Answer from the drawing. Dimensions are ordinates in mm from the lowest x, y and z of the part. A direction names the side the tool comes from. Round coordinates to 2 decimals unless told otherwise and drop trailing zeros. Loops run counter-clockwise (first coordinate to the right, second up) from the corner with the lowest first, then second, coordinate; pieces in that order, holes last. Notation, with made-up numbers: M -36,54 L -3,54 A24 cw -3,83 Z; hole C 72.5,19 d3. An arc over 180 degrees is marked long. One line per item, written item: value.
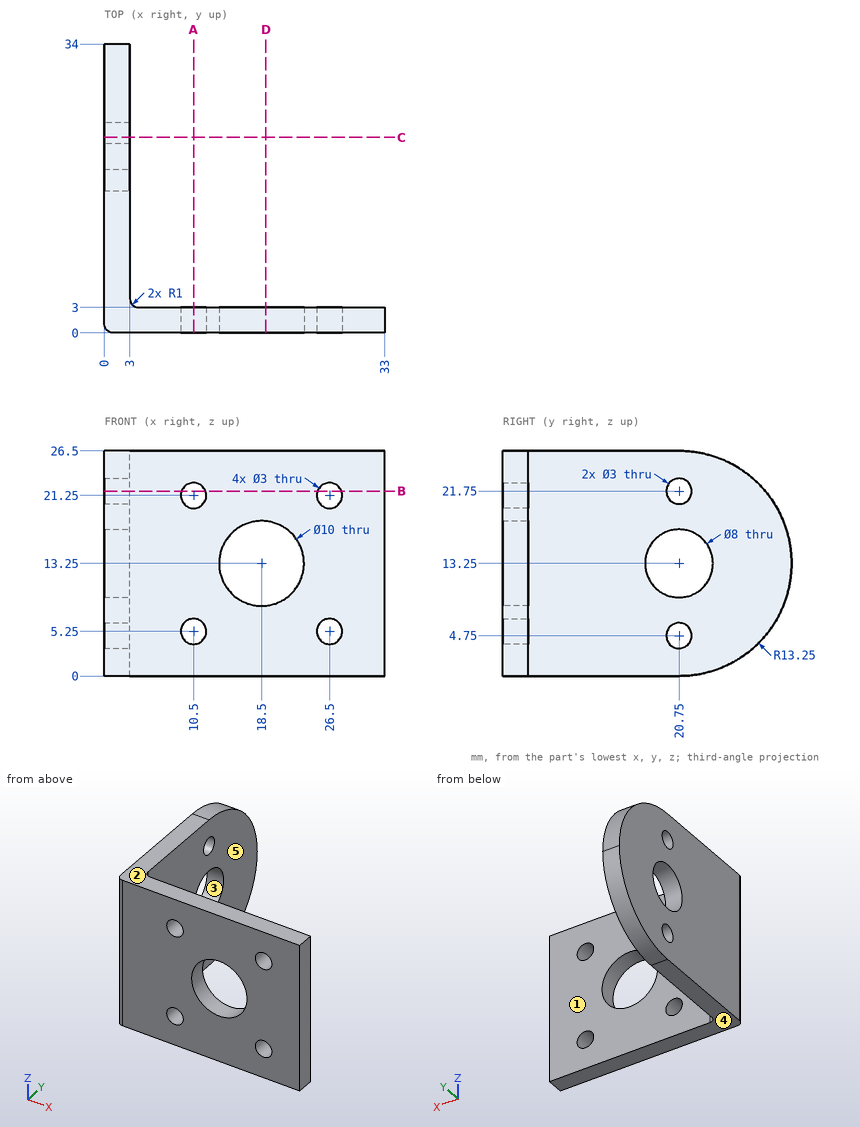
1) Find section B-B (z = 21.75). Give the vertices of the cut face in (x, y).
Check values:
outline: M 0,1 A1 ccw 1,0 L 9.09,0 L 9.09,3 L 4,3 A1 cw 3,4 L 3,19.25 L 0,19.25 Z; M 0,22.25 L 3,22.25 L 3,30.91 L 0,30.91 Z; M 11.91,0 L 25.09,0 L 25.09,3 L 11.91,3 Z; M 27.91,0 L 33,0 L 33,3 L 27.91,3 Z
2) Find section D-D (x = 19). Give the vertices of the cut face in (y, z).
Check values:
outline: M 0,0 L 3,0 L 3,8.28 L 0,8.28 Z; M 0,18.22 L 3,18.22 L 3,26.5 L 0,26.5 Z
3) For the marked faces 4 and 5, determine the directions among +Z, -Z, +X, -X, +Y, -Y from which every point of the face is accessible in a straight line to the end or side of a thin tool.
Check values:
face 4: -Z, +X, -X, +Y, -Y
face 5: +Z, -Z, +X, +Y
4) Find the intervals of material crossed by probe 1 along Z at (x, y) = (26.5, 1.6); probe 2 along X at (y, z) = (1.25, 5.25); probe 3 along Z at (x, y) = (0.85, 20.75), in increasing order. Write a range as from..to.
Check values:
probe 1: 0..3.75, 6.75..19.75, 22.75..26.5
probe 2: 0..9, 12..25, 28..33
probe 3: 0..3.25, 6.25..9.25, 17.25..20.25, 23.25..26.5
5) The mould has two halves that part along Z. Classify the marked faces 1, 2 and 3: +Z half, -Z half, draft (parallel to the pull), parting line (faces both ways), or undercut.
Check values:
face 1: draft
face 2: +Z half
face 3: undercut
6) Find section A-A (x = 10.5). Give the vertices of the cut face in (y, z), then the cut area to 3 significant figures.
Check values:
outline: M 0,0 L 3,0 L 3,3.75 L 0,3.75 Z; M 0,6.75 L 3,6.75 L 3,19.75 L 0,19.75 Z; M 0,22.75 L 3,22.75 L 3,26.5 L 0,26.5 Z
area: 61.5 mm2
7) Find section C-C (y = 23). Give the vertices of the cut face in (x, z).
Check values:
outline: M 0,0.19 L 3,0.19 L 3,9.94 L 0,9.94 Z; M 0,16.56 L 3,16.56 L 3,26.31 L 0,26.31 Z
8) Each of these flat-tipped pins is pushed along its axis until it touches: pin 1 (5 mm diameter, centred on x = 26.5, z = 21.25, fed in from +Y); pin 2 (8 mm diameter, centred on y = 14.5, z = 15, fed in from +X); pin 3 (5 mm diameter, centred on y = 20.75, z = 13.25, fed in from +X). Where does it stop, or does it pass through?
Check values:
pin 1: y = 3
pin 2: x = 3
pin 3: through
